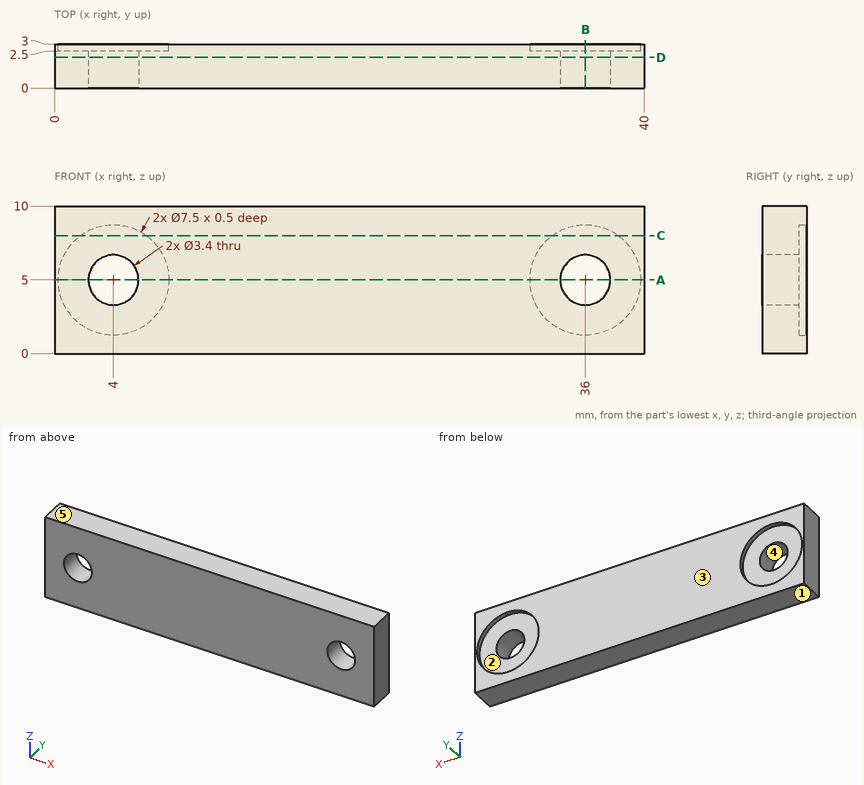
Study the drawing (mm; zero at the part's minimum x, y, z) and answer. A direction names the side the tool comes from. Give positions to 0.01 mm unless a question says otherwise; leave off trailing zeros. Write each loop counter-clockwise with the first axis right and the second up, starting at its lowest first coordinate (ties: lowest second). Pieces come first, ordered by that corner, then holes.
Item 1: Section B-B, the plane x = 36 is taken. Write down the section's boundary in (y, z).
Item 2: Determine the mould class of the marked faces 3, 4 and 5 for opening direction Z: released by +Z, released by -Z, zero draft, split by the parting line, or undercut.
Item 3: Flat-ended cylindrical pins translate along their axes: P1, Ø1, axis at y = 2, z = 8, coming from the -X side; P2, Ø6, axis at x = 4.5, z = 5, coming from the +Y side; P3, Ø2.5, axis at x = 36, z = 5, coming from the -Y side. Find the tip coordinate at first contact, or state that the pin passes through.
Item 4: Section C-C, the plane z = 8 is taken. Write down the section's boundary in (x, y).
Item 5: Section D-D, the plane y = 2.1 is taken. Write down the section's boundary in (x, z), plus the area to 3 significant figures.
Item 6: Find the intervals of material crossed by line 1 along X through (y, z) = (1.35, 5); line 2 along Z through (x, y) = (4, 2.7); line 3 along X through (y, z) = (0.65, 4.25), in increasing order.
Item 7: Which of the six approach directions +Z, -Z, +X, -X, +Y, -Y give full straight-line access (tool end or side, diameter ignored) to the marked faces 1 and 2?
Item 8: Section A-A, the plane z = 5 is taken. Write down the section's boundary in (x, y), plus the area to 3 significant figures.
Completed:
1. outline: (0, 0) - (3, 0) - (3, 1.25) - (2.5, 1.25) - (2.5, 3.3) - (0, 3.3) - close; (0, 6.7) - (2.5, 6.7) - (2.5, 8.75) - (3, 8.75) - (3, 10) - (0, 10) - close
2. face 3: zero draft
2. face 4: undercut
2. face 5: released by +Z
3. P1: stops at x = 0
3. P2: stops at y = 2.5
3. P3: passes through
4. outline: (0, 0) - (40, 0) - (40, 3) - (38.25, 3) - (38.25, 2.5) - (33.75, 2.5) - (33.75, 3) - (6.25, 3) - (6.25, 2.5) - (1.75, 2.5) - (1.75, 3) - (0, 3) - close
5. outline: (0, 0) - (40, 0) - (40, 10) - (0, 10) - close; hole circle Ø3.4 at (4, 5); hole circle Ø3.4 at (36, 5)
5. area: 382 mm2
6. line 1: x = 0 to 2.3, 5.7 to 34.3, 37.7 to 40
6. line 2: z = 0 to 1.25, 8.75 to 10
6. line 3: x = 0 to 2.47, 5.53 to 34.47, 37.53 to 40
7. face 1: -Z, +X, -X, +Y, -Y
7. face 2: +Y
8. outline: (0, 0) - (2.3, 0) - (2.3, 2.5) - (0.25, 2.5) - (0.25, 3) - (0, 3) - close; (5.7, 0) - (34.3, 0) - (34.3, 2.5) - (32.25, 2.5) - (32.25, 3) - (7.75, 3) - (7.75, 2.5) - (5.7, 2.5) - close; (37.7, 0) - (40, 0) - (40, 3) - (39.75, 3) - (39.75, 2.5) - (37.7, 2.5) - close
8. area: 95.5 mm2
